```python
from build123d import *

# Parameters (mm, degrees)
SKETCH_1_R          = 1.625
EXTRUDE_1_DEPTH     = 3
FILLET_1_R          = 10
SKETCH_2_R          = 1.75
CUT_EXTRUDE_1_DEPTH = 10
SKETCH_4_R          = 1.75
CUT_EXTRUDE_2_DEPTH = 10
SKETCH_5_R          = 1.75
CUT_EXTRUDE_3_DEPTH = 10


with BuildPart() as part:
    # Эскиз1 → Бобышка-Вытянуть1 (new body)
    with BuildSketch(Plane.XY):
        with BuildLine():
            ThreePointArc((-32.5, -28.5), (-35.328427125, -35.328427125), (-28.5, -32.5))
            Line((-28.5, -32.5), (28.5, -32.5))
            ThreePointArc((28.5, -32.5), (35.328427125, -35.328427125), (32.5, -28.5))
            Line((32.5, -28.5), (32.5, 28.5))
            ThreePointArc((32.5, 28.5), (35.328427125, 35.328427125), (28.5, 32.5))
            Line((28.5, 32.5), (-28.5, 32.5))
            ThreePointArc((-28.5, 32.5), (-35.328427125, 35.328427125), (-32.5, 28.5))
            Line((-32.5, 28.5), (-32.5, -28.5))
        make_face()
        with Locations((-32.5, -32.5)):
            Circle(SKETCH_1_R, mode=Mode.SUBTRACT)
        with Locations((32.5, 32.5)):
            Circle(SKETCH_1_R, mode=Mode.SUBTRACT)
        with Locations((-32.5, 32.5)):
            Circle(SKETCH_1_R, mode=Mode.SUBTRACT)
        with Locations((32.5, -32.5)):
            Circle(SKETCH_1_R, mode=Mode.SUBTRACT)
    extrude(amount=EXTRUDE_1_DEPTH)

    # Скругление1
    fillet_1_edges = [part.edges().sort_by_distance(p)[0] for p in [
        (-32.5, -28.5, 1.5),
        (-32.5, 28.5, 1.5),
        (-28.5, 32.5, 1.5),
        (28.5, 32.5, 1.5),
        (32.5, 28.5, 1.5),
        (32.5, -28.5, 1.5),
        (28.5, -32.5, 1.5),
        (-28.5, -32.5, 1.5),
    ]]
    fillet(fillet_1_edges, radius=FILLET_1_R)

    # Эскиз2 → Вырез-Вытянуть1 (cut)
    with BuildSketch(Plane.XY.offset(3)):
        with Locations((-13, -25)):
            Circle(SKETCH_2_R)
        with Locations((13, -25)):
            Circle(SKETCH_2_R)
    extrude(amount=-CUT_EXTRUDE_1_DEPTH, mode=Mode.SUBTRACT)

    # Эскиз4 → Вырез-Вытянуть2 (cut)
    with BuildSketch(Plane.XY.offset(3)):
        with Locations((-16.5, -15)):
            Circle(SKETCH_4_R)
        with Locations((16.5, -15)):
            Circle(SKETCH_4_R)
    extrude(amount=-CUT_EXTRUDE_2_DEPTH, mode=Mode.SUBTRACT)

    # Эскиз5 → Вырез-Вытянуть3 (cut)
    with BuildSketch(Plane.XY.offset(3)):
        with Locations((-16.5, 5)):
            Circle(SKETCH_5_R)
        with Locations((16.5, 5)):
            Circle(SKETCH_5_R)
    extrude(amount=-CUT_EXTRUDE_3_DEPTH, mode=Mode.SUBTRACT)


solid = part.part
```
Geometry: final body of the model. Coordinates: model frame, mm. A direction names the side the tool comes from. Round coordinates to 2 decimals unless told otherwise and drop trailing zeros. Order: outer loops, then holes, each group sorted by start corner. A loop starts at its lowest first (then second) coordinate and runs counter-clockwise, first axis right, second up. Notation, with made-up numbers: (65.25, 22) -> (101.25, 22) arc R17 cw to (101.25, 52) -> close; hole circle Ø5 at (-15.75, -32.5). An arc over 180 degrees is marked (long way). Use one line per item in the form item = value. Start each with the question number.
1. Reachability of faces 1 (the face through (33.22, 26.43, 1.52)), 2 (the face through (-33.22, 26.43, 1.52)), 3 (the face through (-26.53, 33.26, 1.52)) from +Z, -Z, +X, -X, +Y, -Y: full face, straight path, thin tool, end or side. Return the list, or none.
2. Cut plane A-A (x = 13). Return the cut outline in (y, z), then the cut area to 4 significant figures.
3. Cut plane B-B (z = 0.45). Count the separate pieces of the cut face and the enclosed holes in it, then the cut area to 3 significant figures.
4. Pin query (flat end, axial travel): pin 1 Ø2.5 at (x, y) = (32.5, 32.5) entering from +Z; pin 2 Ø0.9 at (x, z) = (8.5, 1) entering from -Y; pin 3 Ø1 at (y, z) = (-22, 1.5) entering from +X; pin 4 Ø1.5 at (y, z) = (9.5, 2) entering from -X. Return the tip coordinate at first contact, or that it passes through.
5. Cut plane C-C (y = -15). Return the cut outline in (x, z).
6. Line query: probe 1 along Y at (x, z) = (16.5, 2.45); probe 2 along Y at (x, z) = (-13, 1.05); probe 3 along Y at (x, z) = (-15, 0.35). Output: solid intervals per line, ascending.
7. Draft query along X for faces 4 (the face through (31.302, -31.402, 1.479)), 5 (the face through (32.5, 0, 1)), 6 (the face through (-1, 1, 0)), 7 (the face through (17.31, 3.45, 1.52)). Return one class per face: pulls with the +X half, pulls with the -X half, needs draft (parallel to the pull), parting line crosses it, or undercut.
8. Cut plane D-D (x = -16.5). Return the cut outline in (y, z).
Solution:
q1.face_1 = +Z, -Z, +X
q1.face_2 = +Z, -Z, -X
q1.face_3 = +Z, -Z, +Y
q2.outline = (-32.5, 0) -> (-26.75, 0) -> (-26.75, 3) -> (-32.5, 3) -> close; (-23.25, 0) -> (32.5, 0) -> (32.5, 3) -> (-23.25, 3) -> close
q2.area = 184.5 mm^2
q3.separate_pieces = 1
q3.enclosed_holes = 10
q3.area = 4,320 mm^2
q4.pin_1 = through
q4.pin_2 = -32.5
q4.pin_3 = 32.5
q4.pin_4 = -32.5
q5.outline = (-32.5, 0) -> (-18.25, 0) -> (-18.25, 3) -> (-32.5, 3) -> close; (-14.75, 0) -> (14.75, 0) -> (14.75, 3) -> (-14.75, 3) -> close; (18.25, 0) -> (32.5, 0) -> (32.5, 3) -> (18.25, 3) -> close
q6.probe_1 = -32.5 to -16.75, -13.25 to 3.25, 6.75 to 32.5
q6.probe_2 = -32.5 to -26.75, -23.25 to 32.5
q6.probe_3 = -32.5 to -15.9, -14.1 to 4.1, 5.9 to 32.5
q7.face_4 = undercut
q7.face_5 = pulls with the +X half
q7.face_6 = needs draft
q7.face_7 = undercut
q8.outline = (-32.5, 0) -> (-16.75, 0) -> (-16.75, 3) -> (-32.5, 3) -> close; (-13.25, 0) -> (3.25, 0) -> (3.25, 3) -> (-13.25, 3) -> close; (6.75, 0) -> (32.5, 0) -> (32.5, 3) -> (6.75, 3) -> close
